The listing builds one solid part. Answer for the finished solid, in the listing's coordinates (mm). Give positions to 0.01 mm unless a question says otherwise; leave off trailing zeros. Loops run counter-clockwise (first coordinate to the right, second up) from the corner with the lowest first, then second, coordinate; pieces in that order, holes last. Notation, with made-up numbers: (-33.5, 74.5) - (-25.5, 74.5) arc R18 cw to (-25.5, 107.5) - close; hole circle Ø9 at (0, 78). An arc over 180 degrees is marked (long way). Write item = value, one per line. Start each with the question number.
1) The part is cut by section B-B on x = 87.5. Write down the section's boundary in (y, z), plus the area to 3 significant figures.
2) The part is cut by section C-C on z = 0.7. State how many separate pieces and enclosed holes the cut face has, plus the area to 3 significant figures.
3) The part is cut by section A-A on y = 100. Write down the section's boundary in (x, z).
4) The part is cut by section D-D on y = 33. Write down the section's boundary in (x, z).
5) Consider probe 1 along Y at (x, z) = (87.5, 1.3); probe 2 along Y at (x, z) = (122.5, 0.65); probe 3 along X at (y, z) = (52, 0.35). Determine where each line is inside the solid, lowest interval first.
from build123d import *

# Parameters (mm, degrees)
CROQUIS1_W              = 275
CROQUIS1_H              = 230
CROQUIS1_R              = 3.1
SALIENTE_EXTRUIR1_DEPTH = 3
CROQUIS2_R              = 24.5
CORTAR_EXTRUIR1_DEPTH   = 4
CROQUIS3_R              = 2
CROQUIS3_W              = 25
CROQUIS3_H              = 45
CORTAR_EXTRUIR2_DEPTH   = 4


with BuildPart() as part:
    # Croquis1 → Saliente-Extruir1 (new body)
    with BuildSketch(Plane.XY):
        Rectangle(CROQUIS1_W, CROQUIS1_H)
        with Locations((-122.5, 100)):
            Circle(CROQUIS1_R, mode=Mode.SUBTRACT)
        with Locations((122.275174875, 100)):
            Circle(CROQUIS1_R, mode=Mode.SUBTRACT)
        with Locations((-122.5, -100)):
            Circle(CROQUIS1_R, mode=Mode.SUBTRACT)
        with Locations((122.5, -100)):
            Circle(CROQUIS1_R, mode=Mode.SUBTRACT)
    extrude(amount=SALIENTE_EXTRUIR1_DEPTH)

    # Croquis2 → Cortar-Extruir1 (cut, through all)
    with BuildSketch(Plane.XY.offset(3)):
        with Locations((87.5, 40)):
            Circle(CROQUIS2_R)
        with Locations((87.5, -10)):
            Circle(CROQUIS2_R)
    extrude(amount=-CORTAR_EXTRUIR1_DEPTH, mode=Mode.SUBTRACT)

    # Croquis3 → Cortar-Extruir2 (cut, through all)
    with BuildSketch(Plane.XY.offset(3)):
        with Locations((-112.5, 5)):
            Circle(CROQUIS3_R)
        with Locations((-72.5, 5)):
            Circle(CROQUIS3_R)
        with Locations((-92.5, 5)):
            Rectangle(CROQUIS3_W, CROQUIS3_H)
    extrude(amount=-CORTAR_EXTRUIR2_DEPTH, mode=Mode.SUBTRACT)


solid = part.part
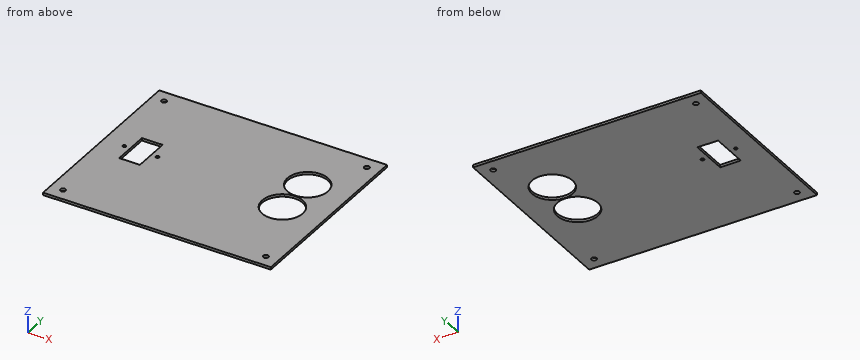
Answer below:
q1.outline = (-115, 0) - (-34.5, 0) - (-34.5, 3) - (-115, 3) - close; (14.5, 0) - (15.5, 0) - (15.5, 3) - (14.5, 3) - close; (64.5, 0) - (115, 0) - (115, 3) - (64.5, 3) - close
q1.area = 396 mm2
q2.separate_pieces = 1
q2.enclosed_holes = 9
q2.area = 58,200 mm2
q3.outline = (-137.5, 0) - (-125.6, 0) - (-125.6, 3) - (-137.5, 3) - close; (-119.4, 0) - (119.18, 0) - (119.18, 3) - (-119.4, 3) - close; (125.38, 0) - (137.5, 0) - (137.5, 3) - (125.38, 3) - close
q4.outline = (-137.5, 0) - (64.02, 0) - (64.02, 3) - (-137.5, 3) - close; (110.98, 0) - (137.5, 0) - (137.5, 3) - (110.98, 3) - close
q5.probe_1 = -115 to -34.5, 14.5 to 15.5, 64.5 to 115
q5.probe_2 = -115 to -103.1, -96.9 to 96.91, 103.09 to 115
q5.probe_3 = -137.5 to 66.14, 108.86 to 137.5
